```python
from build123d import *

# Parameters (mm, degrees)
SKETCH_1_R               = 39
SKETCH_1_R_2             = 29
EXTRUDE_1_DEPTH          = 1.6
SKETCH_2_W               = 3.045590862
SKETCH_2_H               = 7.157138524
EXTRUDE_2_DEPTH          = 1
PATTERN_CIRCULAR_1_COUNT = 18


with BuildPart() as part:
    # 草图1 → 凸台-拉伸1 (new body)
    with BuildSketch(Plane(origin=(0, 0, 0), x_dir=(1, 0, 0), z_dir=(0, 1, 0))):
        with Locations(Location((0, 0, 0), (0, 0, 270))):
            Circle(SKETCH_1_R)
        with Locations(Location((0, 0, 0), (0, 0, 270))):
            Circle(SKETCH_1_R_2, mode=Mode.SUBTRACT)
    extrude(amount=EXTRUDE_1_DEPTH)

    # 草图2 → 凸台-拉伸2 (add)
    with BuildSketch(Plane(origin=(0, 1.6, 0), x_dir=(1, 0, 0), z_dir=(0, 1, 0))):
        with Locations((0, 34.300967075)):
            Rectangle(SKETCH_2_W, SKETCH_2_H)
    extrude_2 = extrude(amount=EXTRUDE_2_DEPTH)

    # 阵列(圆周)1: 凸台-拉伸2 ×18 about axis
    pattern_circular_1_axis = Axis((0, 0, 0), (0, 1, 0))
    for i in range(1, PATTERN_CIRCULAR_1_COUNT):
        add(extrude_2.rotate(pattern_circular_1_axis, i * 360 / PATTERN_CIRCULAR_1_COUNT))


solid = part.part
```
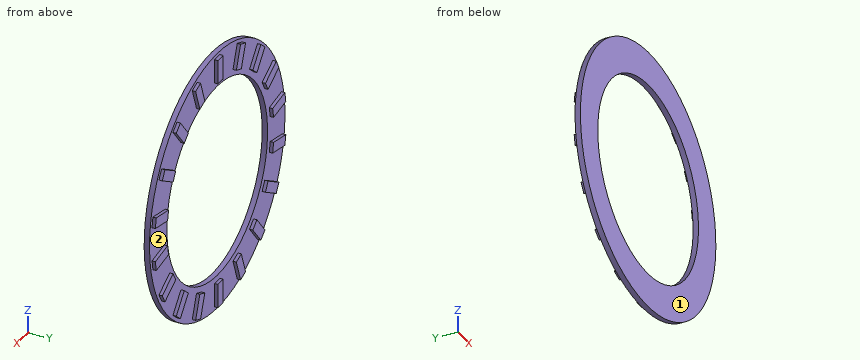
The listing builds one solid part. Answer for the finished solid, in the listing's coordinates (mm). Face numbers are marked on the shaded views. Give positions to 0.01 mm unless a question says otherwise; leave off trailing zeros. Loops run counter-clockwise (first coordinate to the right, second up) from the corner with the lowest first, then second, coordinate; pieces in that order, holes last. Notation, with made-up numbers: M 77,77.5 L 101,77.5 A18 ccw 101,102.5 Z; hole C 18,48 d10. An arc over 180 degrees is marked long. One line per item, written item: value.
Q1. A cutting plane is placed at C-C on y = 2.15. Give the number of separate pieces and of enclosed holes in the cut face, then the cut area to 3 significant figures.
Working result:
separate pieces: 18
enclosed holes: 0
area: 392 mm^2
Q2. Determine the mould class of the marked faces 1 and 2 for opening direction Z: +Z half, -Z half, draft (parallel to the pull), parting line (faces both ways), or undercut.
Working result:
face 1: draft
face 2: undercut
Q3. Flat-ended cylindrical pins translate along their axes: P1, Ø1, axis at x = -22, y = 1.5, coming from the +Z side; P2, Ø0.5, axis at y = 2, z = 35, coming from the +X side; P3, Ø1.1, axis at y = 2, z = -33.5, coming from the -X side. Find the tip coordinate at first contact, or state that the pin passes through.
Working result:
P1: stops at z = 32.54
P2: stops at x = 14.39
P3: stops at x = -20.59
Q4. A cutting plane is placed at D-D on z = -26. Determine the outline of the cut face in (x, y).
Working result:
outline: M -29.07,0 L -12.85,0 L -12.85,1.6 L -19.83,1.6 L -19.83,2.6 L -23.8,2.6 L -23.8,1.6 L -29.07,1.6 Z; M 12.85,0 L 29.07,0 L 29.07,1.6 L 23.8,1.6 L 23.8,2.6 L 19.83,2.6 L 19.83,1.6 L 12.85,1.6 Z
Q5. A cutting plane is placed at B-B on z = 0. Determine the outline of the cut face in (x, y).
Working result:
outline: M -39,0 L -29,0 L -29,1.6 L -39,1.6 Z; M 29,0 L 39,0 L 39,1.6 L 29,1.6 Z
Q6. Find the intervals of material crossed by line 1 (X direction, y = 0.9, z = 0); line 2 (Z direction, x = -31, y = 2.3); line 3 (Z direction, x = 1, y = 2.25), in increasing order. Write a range as from..to.
Working result:
line 1: x = -39..-29, 29..39
line 2: z = -19.66..-16.14, -7.01..-3.92, 3.92..7.01, 16.14..19.66
line 3: z = -37.88..-30.72, 30.72..37.88
Q7. A cutting plane is placed at A-A on x = 0. Determine the outline of the cut face in (y, z), then the cut area to 3 significant figures.
Working result:
outline: M 0,-39 L 1.6,-39 L 1.6,-37.88 L 2.6,-37.88 L 2.6,-30.72 L 1.6,-30.72 L 1.6,-29 L 0,-29 Z; M 0,29 L 1.6,29 L 1.6,30.72 L 2.6,30.72 L 2.6,37.88 L 1.6,37.88 L 1.6,39 L 0,39 Z
area: 46.3 mm^2
